Check sheet for the drawn part. Datum: minimum x, y, z corner. Units: mm. A direction names the side the tool comes from. Coordinates: 2 decimals unless noted, no trailing zeros. Write each loop counter-clockwise with the first axis right and the second up, starting at its lowest first coordinate (ties: lowest second). Pieces come first, ordered by that corner, then holes. Notation, with made-up numbers: M 62,32 L 88,32 A17 cw 88,44 Z; hole C -5.75,81.25 d11. An arc over 180 degrees is marked long. Answer in a Markdown table with one row per item.
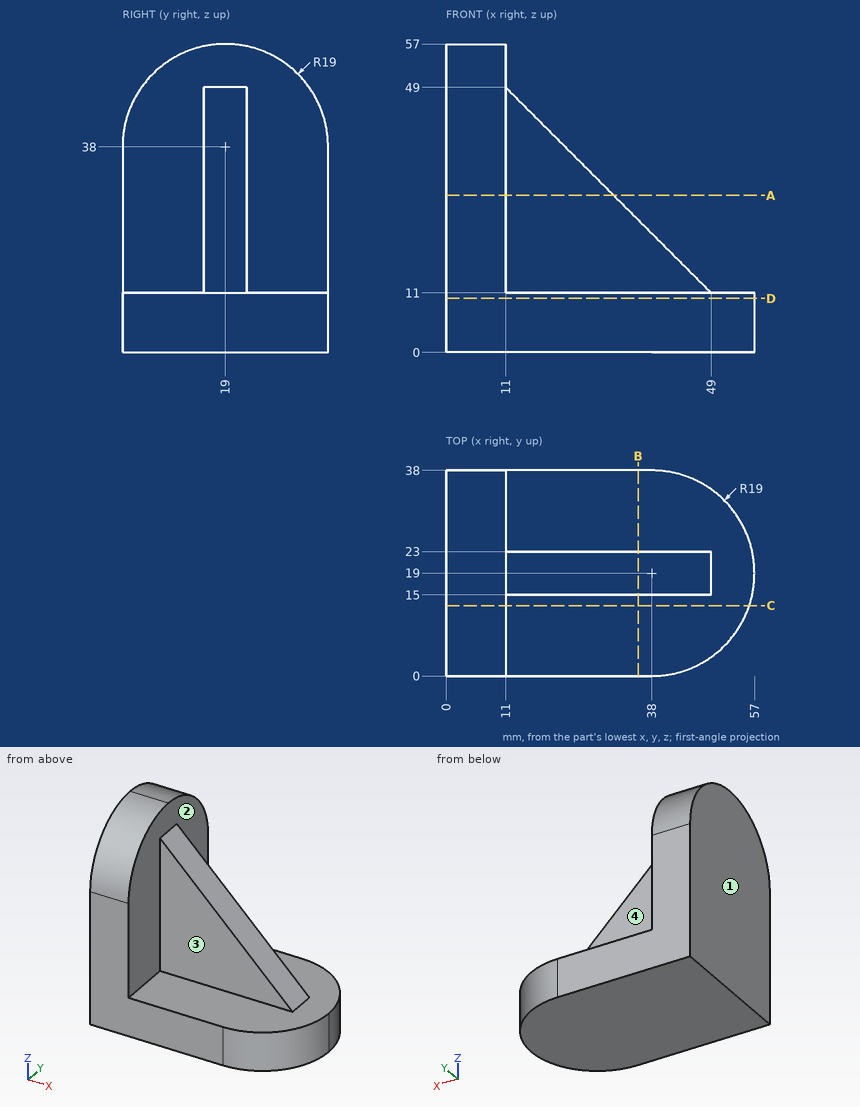
1) Depth check by flat-ended pin: pin 1 (1.5 mm diameter, centred on x = 45.5, y = 9.5, fed in from +Z); pin 2 (1.5 mm diameter, centred on x = 34.5, y = 24, fed in from -Z); pin 3 (3 mm diameter, centred on y = 13, z = 35, fed in from +X); pin 4 (1 mm diameter, centred on x = 26.5, z = 26, fed in from -Y). Enter the tip coordinate at first touch or a pass-through.
Response values:
| item | result |
|---|---|
| pin 1 | stops at z = 11 |
| pin 2 | stops at z = 0 |
| pin 3 | stops at x = 11 |
| pin 4 | stops at y = 15 |
2) Sectioned sample at C-C (y = 13). Record the cut outline in (x, z), then the cut area to 3 significant figures.
Response values:
| item | result |
|---|---|
| outline | M 0,0 L 56.03,0 L 56.03,11 L 11,11 L 11,56.03 L 0,56.03 Z |
| area | 1,110 mm² |
3) Thickness scan on L1, parallel to Z at x = 23, y = 11.5; L2, parallel to Z at x = 37, y = 19.5. Record the ranges inside material, lowest first. Write a range as [from, to].
Response values:
| item | result |
|---|---|
| L1 | z = [0, 11] |
| L2 | z = [0, 23] |
4) Sectioned sample at B-B (x = 35.5). Record the cut outline in (y, z).
Response values:
| item | result |
|---|---|
| outline | M 0,0 L 38,0 L 38,11 L 23,11 L 23,24.5 L 15,24.5 L 15,11 L 0,11 Z |
5) Sectioned sample at A-A (z = 29). Record the cut outline in (x, y), then the cut area to 3 significant figures.
Response values:
| item | result |
|---|---|
| outline | M 0,0 L 11,0 L 11,15 L 31,15 L 31,23 L 11,23 L 11,38 L 0,38 Z |
| area | 578 mm² |
6) Sectioned sample at D-D (z = 10). Record the cut outline in (x, y).
Response values:
| item | result |
|---|---|
| outline | M 0,0 L 38,0 A19 ccw 38,38 L 0,38 Z |
7) Tool access check on the marked faces 1, 2, 3 and 4. Record the directions out of +Z, -Z, +X, -X, +Y, -Y that give a thin tool (end or side, any length) a straight path to the whole face; none if there is none.
Response values:
| item | result |
|---|---|
| face 1 | +Z, -Z, -X, +Y, -Y |
| face 2 | +Z, +X |
| face 3 | +Z, +X, -Y |
| face 4 | +Z, +X, +Y |
